Here's how the part is built. I have some questions about the finished solid (model axes, mm). Face numbers are marked on the shaded views. A direction names the side the tool comes from. Give positions to 0.01 mm unless a question says otherwise; leave off trailing zeros. Loops run counter-clockwise (first coordinate to the right, second up) from the corner with the lowest first, then second, coordinate; pieces in that order, holes last. Notation, with made-up numbers: (-12.75, 29.5) - (43.25, 29.5) arc R28 ccw to (43.25, 67.5) - close; hole circle Ø7 at (-21, 18). An arc over 180 degrees is marked (long way). Return JSON: item names as keys, results as strings. Group by question number.
(1) If we section it at B-B (x = 33.25): Please give me the cut outline in (y, z).
(2) For P1, Ø12, axis at x = -30, y = -26.5, coming from the -Z side; P2, Ø6, axis at x = -39.68, z = -44.89, coming from the +Y side; P3, Ø3, axis at x = -49.68, z = -44.89, coming from the -Y side; P4, Ø4, axis at y = -46.5, z = 3, coming from the +X side, each with a flat end and sliding along its axis, tell me the tip position at first contact or that it passes through.
(3) If we section it at C-C (x = -1.5): Please give me the cut outline in (y, z).
(4) If we section it at D-D (y = -42): Please give me the cut outline in (x, z).
(5) If we section it at A-A (y = 3.5): Please give me the cut outline in (x, z).
(6) On a 3-axis mill with a long thin cutter (end or side, diameter ignored), from which of +Z, -Z, +X, -X, +Y, -Y can I reach the whole of each face in a straight line? I mean the marked faces 1 and 2. Say none if no direction works.
(7) I need wall thicknesses on probe 1 along Y at (x, z) = (-33.25, 5.4); probe 2 along Y at (x, z) = (33, 2); probe 3 along Z at (x, y) = (-33, -10). Which ranges of each line are inside material? Lowest first, please. Write a range as [from, to].
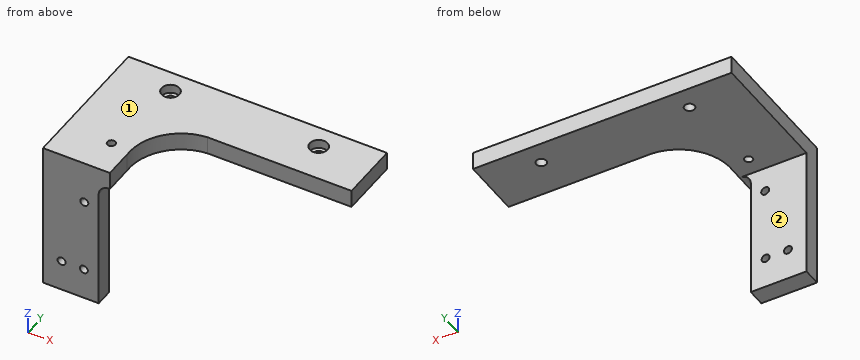
```python
from build123d import *

# Parameters (mm, degrees)
SKETCH_1_R          = 1.8
EXTRUDE_1_DEPTH     = 8
SKETCH_3_R          = 2.25
CUT_EXTRUDE_1_DEPTH = 9
SKETCH_5_R          = 1.8
EXTRUDE_3_DEPTH     = 8
SKETCH_17_R         = 1.8
CUT_EXTRUDE_8_DEPTH = 10
SKETCH_18_R         = 4
CUT_EXTRUDE_9_DEPTH = 4


with BuildPart() as part:
    # 草图1 → 凸台-拉伸1 (new body)
    with BuildSketch(Plane.XY):
        with BuildLine():
            Line((58, 13.5), (58, -13.5))
            Line((58, -13.5), (-6.5, -13.5))
            ThreePointArc((-6.5, -13.5), (-22.42766953, -21.547204204), (-28, -38.5))
            Line((-28, -38.5), (-28, -43.5))
            Line((-28, -43.5), (-58, -43.5))
            Line((-58, -43.5), (-58, 13.5))
            Line((-58, 13.5), (58, 13.5))
        make_face()
        with Locations((-36.769098454, -35.48436381)):
            Circle(SKETCH_1_R, mode=Mode.SUBTRACT)
    extrude(amount=EXTRUDE_1_DEPTH)

    # 草图3 → 切除-拉伸1 (cut, through all)
    with BuildSketch(Plane.XY.offset(8)):
        with Locations((-33.25, 3.5)):
            Circle(SKETCH_3_R)
        with Locations((33.25, 3.5)):
            Circle(SKETCH_3_R)
    extrude(amount=-CUT_EXTRUDE_1_DEPTH, mode=Mode.SUBTRACT)

    # 草图5 → 凸台-拉伸3 (add)
    with BuildSketch(Plane.XZ.offset(43.5)):
        with BuildLine():
            Line((-33, -59), (-58, -59))
            Line((-58, -59), (-58, 8))
            Line((-58, 8), (-28, 8))
            Line((-28, 8), (-28, 0))
            ThreePointArc((-28, 0), (-31.434237008, -1.219913748), (-33, -4.510895309))
            Line((-33, -4.510895309), (-33, -59))
        make_face()
        with Locations((-49.676985034, -44.88768769)):
            Circle(SKETCH_5_R, mode=Mode.SUBTRACT)
        with Locations((-39.676985034, -44.88768769)):
            Circle(SKETCH_5_R, mode=Mode.SUBTRACT)
    extrude(amount=EXTRUDE_3_DEPTH)

    # 草图17 → 切除-拉伸8 (cut)
    with BuildSketch(Plane.XZ.offset(51.5)):
        with Locations((-39.481532593, -11.284064148)):
            Circle(SKETCH_17_R)
    extrude(amount=-CUT_EXTRUDE_8_DEPTH, mode=Mode.SUBTRACT)

    # 草图18 → 切除-拉伸9 (cut)
    with BuildSketch(Plane.XY.offset(8)):
        with Locations((-33.25, 3.5)):
            Circle(SKETCH_18_R)
        with Locations((33.25, 3.5)):
            Circle(SKETCH_18_R)
    extrude(amount=-CUT_EXTRUDE_9_DEPTH, mode=Mode.SUBTRACT)


solid = part.part
```
Values:
{
 "1": {"outline": "(-13.5, 0) - (1.25, 0) - (1.25, 4) - (-0.5, 4) - (-0.5, 8) - (-13.5, 8) - close; (5.75, 0) - (13.5, 0) - (13.5, 8) - (7.5, 8) - (7.5, 4) - (5.75, 4) - close"},
 "2": {"P1": "z = 0", "P2": "y = -43.5", "P3": "through", "P4": "x = -28"},
 "3": {"outline": "(-13.5, 0) - (13.5, 0) - (13.5, 8) - (-13.5, 8) - close"},
 "4": {"outline": "(-58, 0) - (-28, 0) - (-28, 8) - (-58, 8) - close"},
 "5": {"outline": "(-58, 0) - (-35.5, 0) - (-35.5, 4) - (-37.25, 4) - (-37.25, 8) - (-58, 8) - close; (-31, 0) - (31, 0) - (31, 4) - (29.25, 4) - (29.25, 8) - (-29.25, 8) - (-29.25, 4) - (-31, 4) - close; (35.5, 0) - (58, 0) - (58, 8) - (37.25, 8) - (37.25, 4) - (35.5, 4) - close"},
 "6": {"face 1": "+Z, +X, -X, +Y, -Y", "face 2": "-Z, +X, -X, +Y"},
 "7": {"probe 1": "[-51.5, -0.5], [7.5, 13.5]", "probe 2": "[-13.5, 1.26], [5.74, 13.5]", "probe 3": "[0, 8]"}
}
